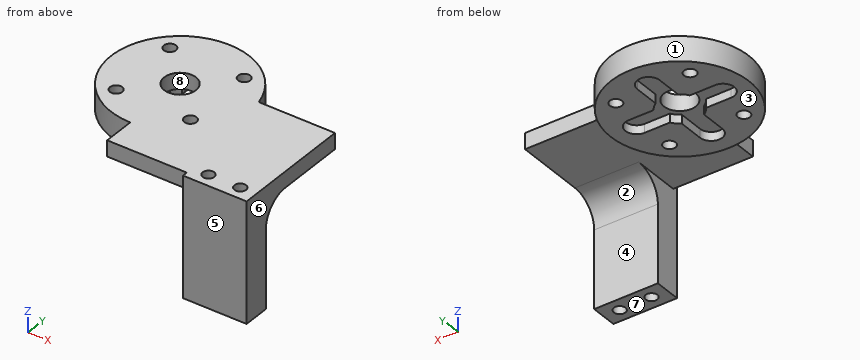
from build123d import *

# Parameters (mm, degrees)
STOCK_HORN_ATTACHMENT_START          = 19.6
STOCK_HORN_ATTACHMENT_PROFILE_R      = 13
STOCK_HORN_ATTACHMENT_DEPTH          = 3
FINGER_ARM_START                     = 19.6
FINGER_ARM_PROFILE_W                 = 27
FINGER_ARM_PROFILE_H                 = 22
FINGER_ARM_DEPTH                     = 3
DESCENDING_CONTACT_FINGER_PROFILE_W  = 12
DESCENDING_CONTACT_FINGER_PROFILE_H  = 5
DESCENDING_CONTACT_FINGER_DEPTH      = 22.6
HORN_CENTER_ACCESS_START             = -50
HORN_CENTER_ACCESS_PROFILE_R         = 3
HORN_CENTER_ACCESS_DEPTH             = 91.493950165
CAPTURED_HORN_KEY_BOSS_START         = 17.95
CAPTURED_HORN_KEY_BOSS_PROFILE_R     = 13
CAPTURED_HORN_KEY_BOSS_DEPTH         = 1.65
KEY_POCKET_HUB_START                 = 17.95
STOCK_HORN_POCKET_HUB_R              = 3.55
KEY_POCKET_HUB_DEPTH                 = 1.65
KEY_POCKET_HORIZONTAL_START          = 17.95
STOCK_HORN_POCKET_HORIZONTAL_W       = 16.3
STOCK_HORN_POCKET_HORIZONTAL_H       = 4.2
KEY_POCKET_HORIZONTAL_DEPTH          = 1.65
KEY_POCKET_VERTICAL_START            = 17.95
STOCK_HORN_POCKET_VERTICAL_W         = 4.2
STOCK_HORN_POCKET_VERTICAL_H         = 16.3
KEY_POCKET_VERTICAL_DEPTH            = 1.65
KEY_POCKET_ROUNDED_TIPS_START        = 17.95
STOCK_HORN_POCKET_ROUNDED_TIPS_R     = 2.1
KEY_POCKET_ROUNDED_TIPS_DEPTH        = 1.65
UNMODIFIED_HORN_CAPTURE_M2_START     = -50
UNMODIFIED_HORN_CAPTURE_M2_PROFILE_R = 1.15
UNMODIFIED_HORN_CAPTURE_M2_DEPTH     = 91.493950165
HUB_CLEARANCE_IN_KEY_BOSS_ONLY_START = 17.95
HORN_CENTER_HUB_CLEARANCE_R          = 4
HUB_CLEARANCE_IN_KEY_BOSS_ONLY_DEPTH = 1.65
CONTACT_PAD_KEEPER_START             = -50
CONTACT_PAD_KEEPER_PROFILE_R         = 1.1
CONTACT_PAD_KEEPER_DEPTH             = 91.493950165
FILLET1_R                            = 5


with BuildPart() as part:
    # Stock_horn_attachment_profile → Stock_horn_attachment (new body)
    with BuildSketch(Plane.XY.offset(STOCK_HORN_ATTACHMENT_START)):
        Circle(STOCK_HORN_ATTACHMENT_PROFILE_R)
    extrude(amount=STOCK_HORN_ATTACHMENT_DEPTH)

    # Finger_arm_profile → Finger_arm (add)
    with BuildSketch(Plane.XY.offset(FINGER_ARM_START)):
        with Locations((13.5, -8)):
            Rectangle(FINGER_ARM_PROFILE_W, FINGER_ARM_PROFILE_H)
    extrude(amount=FINGER_ARM_DEPTH)

    # Descending_contact_finger_profile → Descending_contact_finger (add)
    with BuildSketch(Plane.XY):
        with Locations((21, -17.5)):
            Rectangle(DESCENDING_CONTACT_FINGER_PROFILE_W, DESCENDING_CONTACT_FINGER_PROFILE_H)
    extrude(amount=DESCENDING_CONTACT_FINGER_DEPTH)

    # Horn_center_access_profile → Horn_center_access (cut, through all)
    with BuildSketch(Plane.XY.offset(HORN_CENTER_ACCESS_START)):
        Circle(HORN_CENTER_ACCESS_PROFILE_R)
    extrude(amount=HORN_CENTER_ACCESS_DEPTH, mode=Mode.SUBTRACT)

    # Captured_horn_key_boss_profile → Captured_horn_key_boss (add)
    with BuildSketch(Plane.XY.offset(CAPTURED_HORN_KEY_BOSS_START)):
        with Locations(Location((0, 0, 0), (0, 0, 270))):
            Circle(CAPTURED_HORN_KEY_BOSS_PROFILE_R)
    extrude(amount=CAPTURED_HORN_KEY_BOSS_DEPTH)

    # Stock_horn_pocket_Hub → Key_pocket_Hub (cut)
    with BuildSketch(Plane.XY.offset(KEY_POCKET_HUB_START)):
        Circle(STOCK_HORN_POCKET_HUB_R)
    extrude(amount=KEY_POCKET_HUB_DEPTH, mode=Mode.SUBTRACT)

    # Stock_horn_pocket_Horizontal → Key_pocket_Horizontal (cut)
    with BuildSketch(Plane.XY.offset(KEY_POCKET_HORIZONTAL_START)):
        Rectangle(STOCK_HORN_POCKET_HORIZONTAL_W, STOCK_HORN_POCKET_HORIZONTAL_H)
    extrude(amount=KEY_POCKET_HORIZONTAL_DEPTH, mode=Mode.SUBTRACT)

    # Stock_horn_pocket_Vertical → Key_pocket_Vertical (cut)
    with BuildSketch(Plane.XY.offset(KEY_POCKET_VERTICAL_START)):
        Rectangle(STOCK_HORN_POCKET_VERTICAL_W, STOCK_HORN_POCKET_VERTICAL_H)
    extrude(amount=KEY_POCKET_VERTICAL_DEPTH, mode=Mode.SUBTRACT)

    # Stock_horn_pocket_Rounded_tips → Key_pocket_Rounded_tips (cut)
    with BuildSketch(Plane.XY.offset(KEY_POCKET_ROUNDED_TIPS_START)):
        with Locations((8.15, 0)):
            Circle(STOCK_HORN_POCKET_ROUNDED_TIPS_R)
        with Locations((-8.15, 0)):
            Circle(STOCK_HORN_POCKET_ROUNDED_TIPS_R)
        with Locations((0, 8.15)):
            Circle(STOCK_HORN_POCKET_ROUNDED_TIPS_R)
        with Locations((0, -8.15)):
            Circle(STOCK_HORN_POCKET_ROUNDED_TIPS_R)
    extrude(amount=KEY_POCKET_ROUNDED_TIPS_DEPTH, mode=Mode.SUBTRACT)

    # Unmodified_horn_capture_M2_profile → Unmodified_horn_capture_M2 (cut, through all)
    with BuildSketch(Plane.XY.offset(UNMODIFIED_HORN_CAPTURE_M2_START)):
        with Locations((7, 7)):
            Circle(UNMODIFIED_HORN_CAPTURE_M2_PROFILE_R)
        with Locations((-7, 7)):
            Circle(UNMODIFIED_HORN_CAPTURE_M2_PROFILE_R)
        with Locations((-7, -7)):
            Circle(UNMODIFIED_HORN_CAPTURE_M2_PROFILE_R)
        with Locations((7, -7)):
            Circle(UNMODIFIED_HORN_CAPTURE_M2_PROFILE_R)
    extrude(amount=UNMODIFIED_HORN_CAPTURE_M2_DEPTH, mode=Mode.SUBTRACT)

    # Horn_center_hub_clearance → Hub_clearance_in_key_boss_only (cut)
    with BuildSketch(Plane.XY.offset(HUB_CLEARANCE_IN_KEY_BOSS_ONLY_START)):
        Circle(HORN_CENTER_HUB_CLEARANCE_R)
    extrude(amount=HUB_CLEARANCE_IN_KEY_BOSS_ONLY_DEPTH, mode=Mode.SUBTRACT)

    # Contact_pad_keeper_profile → Contact_pad_keeper (cut, through all)
    with BuildSketch(Plane.XY.offset(CONTACT_PAD_KEEPER_START)):
        with Locations(Location((18, -17.5, 0), (0, 0, 180))):
            Circle(CONTACT_PAD_KEEPER_PROFILE_R)
        with Locations(Location((24, -17.5, 0), (0, 0, 180))):
            Circle(CONTACT_PAD_KEEPER_PROFILE_R)
    extrude(amount=CONTACT_PAD_KEEPER_DEPTH, mode=Mode.SUBTRACT)

    # Fillet1
    fillet1_edges = [part.edges().sort_by_distance(p)[0] for p in [
        (21, -15, 19.6),
    ]]
    fillet(fillet1_edges, radius=FILLET1_R)


solid = part.part
Here's how the part is built. I have some questions about the finished solid (model axes, mm). Face numbers are marked on the shaded views. A direction names the side the tool comes from. Round coordinates to 2 decimals unless told otherwise and drop trailing zeros. Order: outer loops, then holes, each group sorted by start corner. A loop starts at its lowest first (then second) coordinate and runs counter-clockwise, first axis right, second up. Notation, with made-up numbers: M 11.5,-8.5 L 38.5,-8.5 A12 cw 38.5,8.5 Z; hole C 86.25,-2 d5. An arc over 180 degrees is marked long. Return JSON: item names as keys, results as strings. Group by question number.
1. If we mould it in two halves opening along X, with no side actions, what happens to the marked faces 6, 7 and 8? For each: pulls with the +X half, pulls with the -X half, needs draft (parallel to the pull), parting line crosses it, or undercut.
2. If we section it at C-C on y = 0: List the corners of the cut face in (x, z) for me.
3. I'm going to push flat-ended pins straight in: pin 1 Ø1.5 at (x, z) = (18.5, 21.5) entering from +Y; pin 2 Ø3 at (y, z) = (-15, 9.5) entering from -X; pin 3 Ø0.8 at (x, z) = (7, 18.5) entering from -Y. Where does each tip first touch, or does it pass through?
4. On a 3-axis mill with a long thin cutter (end or side, diameter ignored), from which of +Z, -Z, +X, -X, +Y, -Y can I reach the whole of each face in a straight line? I mean the marked faces 1, 2, 3, 4 and 5. Say none if no direction works.
5. If we section it at D-D on x = 7: List the corners of the cut face in (y, z) for me.
6. If we section it at A-A on y = -17.5: List the corners of the cut face in (x, z) for me, then the cut area to 3 significant figures.
7. Please list where these lines run through material, in increasing order: probe 1 along X at (y, z) = (-7, 19.1); probe 2 along X at (y, z) = (7, 19.85).
8. If we section it at B-B on x = 18: List the corners of the cut face in (y, z) for me, then the cut area to 3 significant figures.
Reply:
{
 "1": {"face 6": "pulls with the +X half", "face 7": "needs draft", "face 8": "undercut"},
 "2": {"outline": "M -13,17.95 L -10.25,17.95 L -10.25,19.6 L -3,19.6 L -3,22.6 L -13,22.6 Z; M 3,19.6 L 10.25,19.6 L 10.25,17.95 L 13,17.95 L 13,19.6 L 27,19.6 L 27,22.6 L 3,22.6 Z"},
 "3": {"pin 1": "y = 3", "pin 2": "x = 15", "pin 3": "y = -11.2"},
 "4": {"face 1": "-Z", "face 2": "-Z, +X, +Y", "face 3": "-Z, +X, -X, +Y, -Y", "face 4": "-Z, +X, -X, +Y", "face 5": "+Z, -Z, +X, -X, -Y"},
 "5": {"outline": "M -19,19.6 L -10.95,19.6 L -10.95,17.95 L -8.15,17.95 L -8.15,22.6 L -19,22.6 Z; M -5.85,17.95 L -2.1,17.95 L -2.1,19.6 L 2.1,19.6 L 2.1,17.95 L 5.85,17.95 L 5.85,22.6 L -5.85,22.6 Z; M 8.15,17.95 L 10.95,17.95 L 10.95,22.6 L 8.15,22.6 Z"},
 "6": {"outline": "M 0,19.6 L 15,19.6 L 15,0 L 16.9,0 L 16.9,22.6 L 0,22.6 Z; M 19.1,0 L 22.9,0 L 22.9,22.6 L 19.1,22.6 Z; M 25.1,0 L 27,0 L 27,22.6 L 25.1,22.6 Z", "area": "217 mm^2"},
 "7": {"probe 1": "-10.95 to -8.15, -5.85 to -2.1, 2.1 to 5.85, 8.15 to 10.95", "probe 2": "-10.95 to -8.15, -5.85 to 5.85, 8.15 to 10.95"},
 "8": {"outline": "M -20,0 L -18.6,0 L -18.6,22.6 L -20,22.6 Z; M -16.4,0 L -15,0 L -15,14.6 A5 cw -10,19.6 L 3,19.6 L 3,22.6 L -16.4,22.6 Z", "area": "123 mm^2"}
}
